from build123d import *

# Parameters (mm, degrees)
F5_W         = 64
F5_H         = 45.8
F5_W_2       = 59.2
F5_H_2       = 41
F6_DEPTH     = 24.7
F7_W         = 64
F7_H         = 45.8
F7_W_2       = 59.2
F7_H_2       = 41
F8_DEPTH     = 2.4
F9_R         = 5
F10_DEPTH    = 1.9
F11_R        = 14.82
F11_R_2      = 12.42
F12_DEPTH    = 4
F13_DEPTH    = 1.9
F14_R        = 5
F15_DEPTH    = 2.4
F17_R        = 1.75
F18_DEPTH    = 2.4
F20_DEPTH    = 2.4
F22_DEPTH    = 2.4
F23_R        = 1.75
F24_REACH    = 60.3061382673
F25_R        = 0.5
F26_W        = 18
F26_H        = 2.4
F27_DEPTH    = 24.7
F28_R        = 3.75
F29_REACH    = 63.5629925168
F31_DEPTH    = 2.4
F32_T1_DEPTH = 2.4


# Not quite as in the source:
# - a fillet or chamfer that OpenCascade refuses, or shapes differently, is made with other operations: its cross-section is extruded or revolved along the edge and cut away or added
# - a feature names something its author has since deleted; it is built from what else it names


with BuildPart() as f6:
    # F5 (on Top) → F6 (new body)
    with BuildSketch(Plane.XY):
        Rectangle(F5_W, F5_H)
        Rectangle(F5_W_2, F5_H_2, mode=Mode.SUBTRACT)
    extrude(amount=F6_DEPTH)

    # F7 (on face) → F8 (join)
    with BuildSketch(Plane.XY.offset(24.7)):
        Rectangle(F7_W, F7_H)
        Rectangle(F7_W_2, F7_H_2, mode=Mode.SUBTRACT)
        Rectangle(F7_W_2, F7_H_2)
    extrude(amount=F8_DEPTH)

    # F9 (on face) → F10 (cut)
    with BuildSketch(Plane.XY.offset(27.1)):
        with Locations((-18.6, 7.5)):
            Circle(F9_R)
    extrude(amount=-F10_DEPTH, mode=Mode.SUBTRACT)

    # F11 (on face) → F12 (join)
    with BuildSketch(Plane.XY.offset(27.1)):
        with Locations((13.926, 5.264)):
            Circle(F11_R)
        with Locations((13.926, 5.264)):
            Circle(F11_R_2, mode=Mode.SUBTRACT)
    extrude(amount=F12_DEPTH)

    # F13 (cut): a face of the model
    f13_faces = [f6.faces().sort_by_distance(p)[0] for p in [
        (13.926, 5.264, 27.1),
    ]]
    extrude(f13_faces, amount=-F13_DEPTH, mode=Mode.SUBTRACT)

    # F14 (on face) → F15 (cut)
    with BuildSketch(Plane(origin=(0, 22.9, 0), x_dir=(-1, 0, 0), z_dir=(0, 1, 0))):
        with Locations((17.1, 13.55)):
            Circle(F14_R)
    extrude(amount=-F15_DEPTH, mode=Mode.SUBTRACT)

    # F17 (on face) → F18 (join)
    with BuildSketch(Plane(origin=(0, -15.3661306411, -10.759480508), x_dir=(-1, 0, 0), z_dir=(0, 0.8191520443, 0.5735764364))):
        Polygon((0, 24.1349003924), (0, 13.1349003924), (21, 13.1349003924), (21, 35.1349003924), (0, 35.1349003924), align=None)
        with Locations((16.25, 30.1349003924)):
            Circle(F17_R, mode=Mode.SUBTRACT)
        Polygon((-21, 13.1349003924), (0, 13.1349003924), (0, 24.1349003924), (0, 35.1349003924), (-21, 35.1349003924), align=None)
        with Locations((-16.25, 30.1349003924)):
            Circle(F17_R, mode=Mode.SUBTRACT)
    extrude(amount=F18_DEPTH)

    # F19 (on face) → F20 (join)
    with BuildSketch(Plane(origin=(-21, 0, 0), x_dir=(0, -1, 0), z_dir=(-1, 0, 0))):
        Polygon((22.9, 0), (35.5186815997, 18.0213449744), (33.5527166934, 19.3979284216), (22.9, 19.3979284216), align=None)
    extrude(amount=F20_DEPTH)

    # F21 (on face) → F22 (join)
    with BuildSketch(Plane.YZ.offset(21)):
        Polygon((-35.5186815997, 18.0213449744), (-22.9, 0), (-22.9, 19.3979284216), (-33.5527166934, 19.3979284216), align=None)
    extrude(amount=F22_DEPTH)

    f24_end = f6.faces().sort_by_distance((0, 0, 24.7))[0]
    # F23 (on face) → F24 (cut, up to a face of the model that its end follows)
    with BuildSketch(Plane(origin=(0, -15.3661306411, -10.759480508), x_dir=(1, 0, 0), z_dir=(0, -0.8191520443, -0.5735764364))):
        with Locations((-16.25, 30.1349003924)):
            Circle(F23_R)
        with Locations((16.25, 30.1349003924)):
            Circle(F23_R)
    f24_long = extrude(amount=-F24_REACH, mode=Mode.PRIVATE)
    add(split(f24_long, bisect_by=f24_end, keep=Keep.TOP, mode=Mode.PRIVATE), mode=Mode.SUBTRACT)

    # F25
    f25_edges = [f6.edges().sort_by_distance(p)[0] for p in [
        (-32, 0, 27.1),
        (0, -22.9, 27.1),
        (32, 0, 27.1),
        (0, 22.9, 27.1),
        (-23.6, 7.5, 27.1),
        (32, 0, 0),
        (0, 22.9, 0),
        (-32, 22.9, 13.55),
        (-32, 0, 0),
        (-32, -22.9, 13.55),
        (32, -22.9, 13.55),
    ]]
    fillet(f25_edges, radius=F25_R)

    # F26 (on face) → F27 (cut, through all)
    with BuildSketch(Plane(origin=(0, 0, 0), x_dir=(1, 0, 0), z_dir=(0, 0, -1))):
        with Locations((0, 21.7)):
            Rectangle(F26_W, F26_H)
    extrude(amount=-F27_DEPTH, mode=Mode.SUBTRACT)

    f29_end = Plane(origin=(0, -0.3794689119, 24.7), x_dir=(-1, 0, 0), z_dir=(0, 0, -1))
    # F28 (on face) → F29 (cut, up to a plane its end follows)
    with BuildSketch(Plane(origin=(0, -13.4001657348, -9.3828970608), x_dir=(-1, 0, 0), z_dir=(0, 0.8191520443, 0.5735764364))):
        with Locations((16.25, 30.1349003924)):
            Circle(F28_R)
        with Locations((-16.25, 30.1349003924)):
            Circle(F28_R)
    f29_long = extrude(amount=F29_REACH, mode=Mode.PRIVATE)
    add(split(f29_long, bisect_by=f29_end, keep=Keep.TOP, mode=Mode.PRIVATE), mode=Mode.SUBTRACT)

    # F30 (on face) → F31 (cut)
    with BuildSketch(Plane(origin=(0, -15.3661306411, -10.759480508), x_dir=(1, 0, 0), z_dir=(0, -0.8191520443, -0.5735764364))):
        Polygon((12.5, 28.3849003924), (-12.5, 28.3849003924), (-12.5, 15.1349003924), (0, 15.1349003924), (12.5, 15.1349003924), align=None)
    extrude(amount=-F31_DEPTH, mode=Mode.SUBTRACT)

    # F32: fillet of radius 2 on 2 edges, made by hand

    # F32_s2 → F32_t1 (join)
    with BuildSketch(Plane(origin=(0, -15.3661306411, -10.759480508), x_dir=(1, 0, 0), z_dir=(0, 0.8191520443, 0.5735764364))):
        with BuildLine():
            ThreePointArc((-10.5, -15.1349003924), (-11.9142135624, -15.7206868301), (-12.5, -17.1349003924))
            Line((-12.5, -17.1349003924), (-12.5, -15.1349003924))
            Line((-12.5, -15.1349003924), (-10.5, -15.1349003924))
        make_face()
        with BuildLine():
            ThreePointArc((12.5, -17.1349003924), (11.9142135624, -15.7206868301), (10.5, -15.1349003924))
            Line((10.5, -15.1349003924), (12.5, -15.1349003924))
            Line((12.5, -15.1349003924), (12.5, -17.1349003924))
        make_face()
    extrude(amount=F32_T1_DEPTH)


solid = f6.part
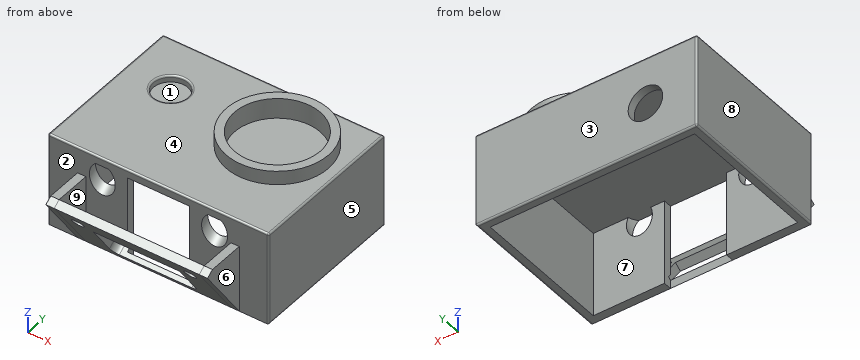
Part model, mm, in its own coordinate system. Face numbers are marked on the shaded views. A direction names the side the tool comes from. Give positions to 0.01 mm unless a question says otherwise; leave off trailing zeros. Loops run counter-clockwise (first coordinate to the right, second up) from the corner with the lowest first, then second, coordinate; pieces in that order, holes last. Notation, with made-up numbers: (65.5, -22) -> (115.5, -22) arc R19 cw to (115.5, 1) -> close; hole circle Ø1 at (64, -32). An arc over 180 degrees is marked (long way). Write each question's results on one line, items separated by ' | '. Start each with the question number.
Q1. Band-saw the part on A-A on x = -2. List the corners of the cut face in (y, z), plus the area to 3 significant figures.
Q2. Wall check: L1, parallel to Y at x = -26.5, z = 22.5; L2, parallel to X at y = 16.5, z = 18; L3, parallel to X at y = -24.5, z = 13. Give the ranges that are in metal, low to high.
Q3. Pull direction Y, two halves, no side cores. Call the marked faces 1, 2, 3 and 4: +Y half, -Y half, draft (parallel to the pull), parting line (faces both ways), or undercut.
Q4. Which spindle directions (+Z, -Z, +X, -X, +Y, -Y) get a long thin tool onto all of the face, cutting with end or side? Do the marked faces 5, 6, 7, 8 and 9. Say none if no direction does.
Q5. Band-saw the part on C-C on y = 1. List the corners of the cut face in (x, z).
Q6. Band-saw the part on D-D on x = 7. List the corners of the cut face in (y, z), plus the area to 3 significant figures.
Q7. Pin check, flat tips, straight feed: P1, Ø1, axis at x = -2, y = 13, coming from the -Z side; P2, Ø6, axis at x = -17.1, z = 13.55, coming from the -Y side; P3, Ø0.7, axis at x = -22, y = -29, coming from the +Z side. Stop position of each tip, or through.
Results are:
1) outline: (-35.52, 18.02) -> (-31.65, 12.49) -> (-29.68, 13.87) -> (-33.55, 19.4) -> close; (-24.05, 1.64) -> (-22.9, 0) -> (-22.9, 2.44) -> close; (-22.9, 24.7) -> (20.5, 24.7) -> (20.5, 0) -> (22.4, 0) arc R0.5 ccw to (22.9, 0.5) -> (22.9, 26.6) arc R0.5 ccw to (22.4, 27.1) -> (-22.4, 27.1) arc R0.5 ccw to (-22.9, 26.6) -> close | area: 187 mm²
2) L1: y = -22.9 to -20.5, 20.5 to 22.9 | L2: x = -32 to -29.6, 29.6 to 32 | L3: x = -23.4 to -21, 21 to 23.4
3) face 1: undercut | face 2: undercut | face 3: +Y half | face 4: draft
4) face 5: +Z, -Z, +X, +Y, -Y | face 6: +Z, -Z, +X, -Y | face 7: -Z | face 8: +Z, -Z, -X, +Y, -Y | face 9: +Z
5) outline: (-32, 0.5) arc R0.5 ccw to (-31.5, 0) -> (-29.6, 0) -> (-29.6, 24.7) -> (29.6, 24.7) -> (29.6, 0) -> (31.5, 0) arc R0.5 ccw to (32, 0.5) -> (32, 26.6) arc R0.5 ccw to (31.5, 27.1) -> (28.12, 27.1) -> (28.12, 31.1) -> (25.59, 31.1) -> (25.59, 25.2) -> (2.26, 25.2) -> (2.26, 31.1) -> (-0.27, 31.1) -> (-0.27, 27.1) -> (-31.5, 27.1) arc R0.5 ccw to (-32, 26.6) -> close
6) outline: (-35.52, 18.02) -> (-31.65, 12.49) -> (-29.68, 13.87) -> (-33.55, 19.4) -> close; (-24.05, 1.64) -> (-22.9, 0) -> (-22.9, 2.44) -> close; (-22.9, 24.7) -> (20.5, 24.7) -> (20.5, 0) -> (22.4, 0) arc R0.5 ccw to (22.9, 0.5) -> (22.9, 26.6) arc R0.5 ccw to (22.4, 27.1) -> (18.37, 27.1) -> (18.37, 31.1) -> (15.57, 31.1) -> (15.57, 25.2) -> (-5.05, 25.2) -> (-5.05, 31.1) -> (-7.84, 31.1) -> (-7.84, 27.1) -> (-22.4, 27.1) arc R0.5 ccw to (-22.9, 26.6) -> close | area: 170 mm²
7) P1: stops at z = 24.7 | P2: stops at y = -34.49 | P3: stops at z = 19.4
